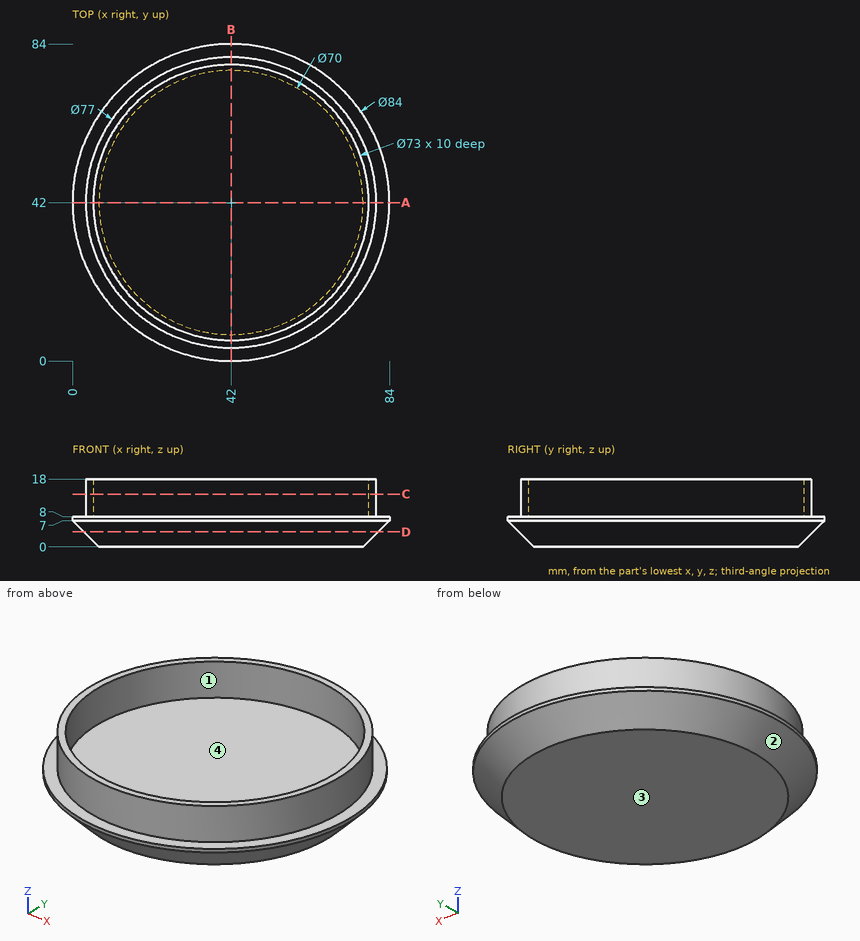
The drawing under review shows one solid part. Ordinate dimensions are in mm from its lowest x, y, z. Coordinates: 2 decimals unless noted, no trailing zeros. Loops run counter-clockwise (first coordinate to the right, second up) from the corner with the lowest first, then second, coordinate; pieces in that order, holes last. Notation, with made-up numbers: M 57,88.25 L 63,88.25 A21 ccw 63,125.25 Z; hole C -10.75,88 d10. An arc over 180 degrees is marked long. Use one line per item in the form item = value.
(1) For line 1 along Y through (x, z) = (42, 14.25); line 2 along Z through (x, y) = (72, 48); line 3 along Y through (x, z) = (75.5, 11), list the stretches that pass through material, from the lowest coordinate up. Write a range as from..to.
Return value:
line_1 = 3.5..5.5, 78.5..80.5
line_2 = 0..8
line_3 = 23.03..27.51, 56.49..60.97
(2) Consider section D-D (z = 4). Write out the cut boundary in (x, y), and give its area (3 significant figures).
Return value:
outline = C 42,42 d78
area = 4,780 mm2
(3) Consider section C-C (z = 14). Write out the cut boundary in (x, y), and give its area (3 significant figures).
Return value:
outline = C 42,42 d77; hole C 42,42 d73
area = 471 mm2
(4) Draft analysis for pull direction X (two halves, no side actions). For the marked faces 1, 2, 3 and 4, state which applies: pulls with the +X half, pulls with the -X half, needs draft (parallel to the pull), parting line crosses it, or undercut.
Return value:
face_1 = undercut
face_2 = parting line crosses it
face_3 = needs draft
face_4 = undercut
(5) Consider section A-A (y = 42). Write out the cut boundary in (x, z).
Return value:
outline = M 0,7 L 7,0 L 77,0 L 84,7 L 84,8 L 80.5,8 L 80.5,18 L 78.5,18 L 78.5,8 L 5.5,8 L 5.5,18 L 3.5,18 L 3.5,8 L 0,8 Z
(6) Clearance check with flat-ended pins moving along their axes: P1, Ø3, axis at y = 73, z = 6, coming from the -X side; P2, Ø1.5, axis at y = 73, z = 9.5, coming from the +X side; P3, Ø5, axis at x = 65.5, z = 2.5, coming from the +Y side. State where each tip first meets the part, or that it passes through.
Return value:
P1 = 12.49
P2 = 65.82
P3 = 74.84
